Job drawing, mm, ordinate dimensions from the low corner. One solid piece. Round coordinates to 2 decimals unless told otherwise and drop trailing zeros. Order: outer loops, then holes, each group sorted by start corner. A loop starts at its lowest first (then second) coordinate and runs counter-clockwise, first axis right, second up. Notation, with made-up numbers: (67, -21) -> (100, -21) arc R8 ccw to (100, -15) -> close; hole circle Ø4 at (2, 22.5). An arc over 180 degrees is marked (long way). Use CSV: the item, a comma, the result in double quotes.
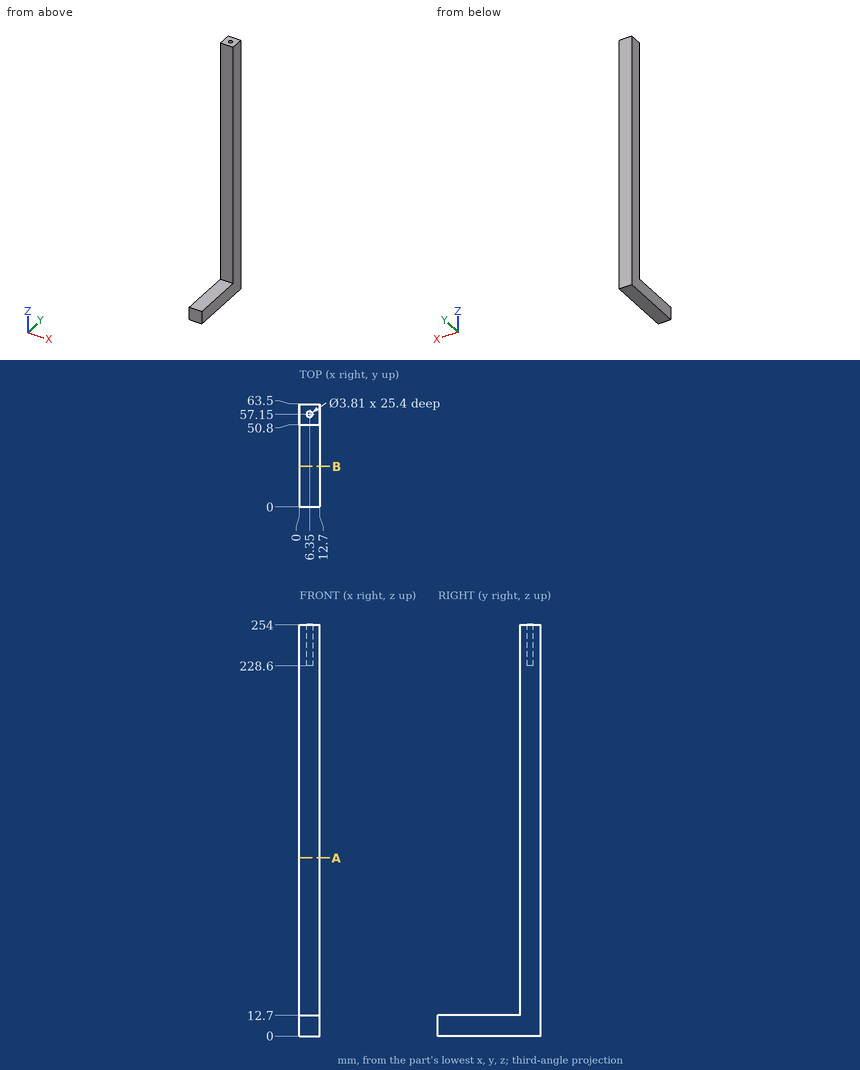
(1) Probe probe 1 along Y at (x, z) = (6.35, 247.75) (3 decimals); probe 2 along X at (y, z) = (57.15, 237.5) (3 decimals); probe 3 along Y at (x, z) = (8, 15.5). List the from-to ranges inside material, lowest first. Write a range as [from, to].
Reply:
probe 1,"[50.8, 55.245], [59.055, 63.5]"
probe 2,"[0, 4.445], [8.255, 12.7]"
probe 3,"[50.8, 63.5]"
(2) Drop flat-ended pins along their axis: P1, Ø1.1, axis at x = 6.5, y = 58, coming from the +Z side; P2, Ø6, axis at x = 10, z = 68, coming from the -Y side. Give the stop position or say it passes through.
Reply:
P1,"z = 228.6"
P2,"y = 50.8"
(3) Cut at B-B, the plane y = 25. Give the cut face in (x, z), then the cut area to 3 significant figures.
Reply:
outline,"(0, 0) -> (12.7, 0) -> (12.7, 12.7) -> (0, 12.7) -> close"
area,"161 mm2"
(4) Cut at A-A, the plane z = 110. Give the cut face in (x, y).
Reply:
outline,"(0, 50.8) -> (12.7, 50.8) -> (12.7, 63.5) -> (0, 63.5) -> close"
